The listing builds one solid part. Answer for the finished solid, in the listing's coordinates (mm). Face numbers are marked on the shaded views. Round coordinates to 2 decimals unless told otherwise and drop trailing zeros. Loops run counter-clockwise (first coordinate to the right, second up) from the corner with the lowest first, then second, coordinate; pieces in that order, holes last. Notation, with made-up numbers: M 73.5,17 L 86.5,17 A19 cw 86.5,23 Z; hole C 25.25,-19 d2. An arc over 180 degrees is marked long. Put each result on its own line as item: value. Start each with the question number.
(1) Section B-B, the plane z = 50 is taken. Determine the outline of the cut face in (x, y).
(2) Flat-ended cylindrical pins translate along their axes: P1, Ø10, axis at y = 1.5, z = 57.5, coming from the +X side (3 decimals); P2, Ø2.5, axis at x = 1.5, y = 12.5, coming from the +Z side; P3, Ø6, axis at x = -0.5, y = 7, coming from the +Z side; P4, Ø1, axis at y = 2, z = 89, coming from the -X side. Find the tip coordinate at first contact, or state that the pin passes through.
(3) Section D-D, the plane x = -20 is taken. Count the separate pieces of the cut face and the enclosed holes in it, then the cut area to 3 significant figures.
(4) Section A-A, the plane x = 1.5 is taken. Determine the outline of the cut face in (y, z), then the cut area to 3 significant figures.
(5) Straight lines are drawn through the part: line 1 (X direction, y = 11.5, z = 94); line 2 (Y direction, x = 0, z = 88.5); line 3 (Z direction, x = -23.5, y = 5.5). For each, find the intervals that lie inside material, in ascending order.
(6) Determine the mould class of the marked faces 1, 2 and 3 for opening direction X: released by +X, released by -X, zero draft, split by the parting line, or undercut.
(7) Section C-C, the plane y = -13 is taken. Determine the outline of the cut face in (x, z).
```python
from build123d import *

# Parameters (mm, degrees)
PAD_DEPTH       = 116
SKETCH001_R     = 1.75
POCKET_DEPTH    = 17.6055143834
SKETCH002_R     = 4
POCKET001_DEPTH = 14
SKETCH003_W     = 20
SKETCH003_H     = 16
POCKET002_DEPTH = 5
FILLET_R        = 2
FILLET001_R     = 2
FILLET002_R     = 0.5
FILLET003_R     = 0.5


with BuildPart() as part:
    # Sketch (on XY_Plane of Origin) → Pad (new body)
    with BuildSketch(Plane.XY):
        Polygon((10.1949841474, 13.6874291489), (-11.9050158526, 13.6874291489), (-27.9319746193, 13.6874291489), (-11.9050158526, -20.6824948412), (10.1949841474, -20.6824948412), (10.1949841474, -18.6824948412), (10.1949841474, -17.3125708511), (8.1949841474, -17.3125708511), (8.1949841474, -18.3125708511), (-9.9050158526, -18.3125708511), (-9.9050158526, 11.6874291489), (8.1949841474, 11.6874291489), (8.1949841474, 10.6874291489), (10.1949841474, 10.6874291489), align=None)
    extrude(amount=PAD_DEPTH)

    # Sketch001 (on Face10 of Pad) → Pocket (cut)
    with BuildSketch(Plane(origin=(-17.7005613893, -8.2539073295, 0), x_dir=(0.4226182617, -0.906307787, 0), z_dir=(-0.906307787, -0.4226182617, 0))):
        with Locations((-16, 109.75)):
            Circle(SKETCH001_R)
        with Locations((-16, 12.25)):
            Circle(SKETCH001_R)
    extrude(amount=-POCKET_DEPTH, mode=Mode.SUBTRACT)

    # Sketch002 (on Face12 of Pocket) → Pocket001 (cut)
    with BuildSketch(Plane(origin=(2.2382099255, 1.0436944288, 0), x_dir=(0.4226182617, -0.906307787, 0), z_dir=(-0.906307787, -0.4226182617, 0))):
        with Locations((-16, 109.75)):
            Circle(SKETCH002_R)
        with Locations((-16, 12.25)):
            Circle(SKETCH002_R)
    extrude(amount=POCKET001_DEPTH, mode=Mode.SUBTRACT)

    # Sketch003 (on Face11 of Pocket001) → Pocket002 (cut)
    with BuildSketch(Plane(origin=(0, 13.6874291489, 0), x_dir=(-1, 0, 0), z_dir=(0, 1, 0))):
        with Locations((-0.1949841474, 8)):
            Rectangle(SKETCH003_W, SKETCH003_H)
        with Locations((-0.1949841474, 108)):
            Rectangle(SKETCH003_W, SKETCH003_H)
    extrude(amount=-POCKET002_DEPTH, mode=Mode.SUBTRACT)

    # Fillet
    fillet_edges = [part.edges().sort_by_distance(p)[0] for p in [
        (-27.931975, 13.687429, 58),
        (-11.905016, -20.682495, 58),
    ]]
    fillet(fillet_edges, radius=FILLET_R)

    # Fillet001
    fillet001_edges = [part.edges().sort_by_distance(p)[0] for p in [
        (10.194984, -20.682495, 58),
        (10.194984, 13.687429, 58),
    ]]
    fillet(fillet001_edges, radius=FILLET001_R)

    # Fillet002
    fillet002_edges = [part.edges().sort_by_distance(p)[0] for p in [
        (8.194984, 10.687429, 58),
        (8.194984, -17.312571, 58),
    ]]
    fillet(fillet002_edges, radius=FILLET002_R)

    # Fillet003
    fillet003_edges = [part.edges().sort_by_distance(p)[0] for p in [
        (10.194984, 10.687429, 58),
        (10.194984, -17.312571, 58),
    ]]
    fillet(fillet003_edges, radius=FILLET003_R)


solid = part.part
```
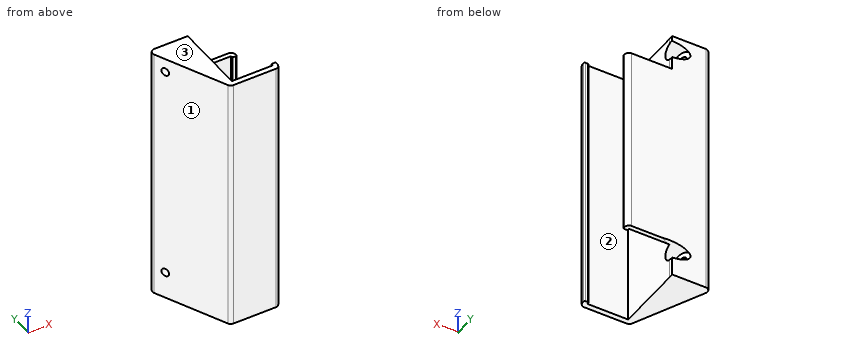
Recorded:
1. outline: M -26.61,10.84 L -12.44,-19.53 A2 ccw -10.63,-20.68 L 8.19,-20.68 A2 ccw 10.19,-18.68 L 10.19,-17.81 A0.5 ccw 9.69,-17.31 L 8.69,-17.31 A0.5 ccw 8.19,-17.81 L 8.19,-18.31 L -9.91,-18.31 L -9.91,11.69 L 8.19,11.69 L 8.19,11.19 A0.5 ccw 8.69,10.69 L 9.69,10.69 A0.5 ccw 10.19,11.19 L 10.19,11.69 A2 ccw 8.19,13.69 L -24.79,13.69 A2 ccw Z
2. P1: stops at x = -9.905
2. P2: stops at z = 100
2. P3: passes through
2. P4: stops at x = -22.72
3. separate pieces: 1
3. enclosed holes: 2
3. area: 1,950 mm²
4. outline: M -20.68,0 L -18.31,0 L -18.31,116 L -20.68,116 Z; M 11.69,16 L 13.69,16 L 13.69,100 L 11.69,100 Z
4. area: 443 mm²
5. line 1: x = -26.78 to -9.91, 8.19 to 10.19
5. line 2: y = -20.68 to -18.31, 11.69 to 13.69
5. line 3: z = 0 to 10.88, 13.62 to 108.38, 111.12 to 116
6. face 1: released by -X
6. face 2: undercut
6. face 3: zero draft
7. outline: M -15.49,0 L -9.91,0 L -9.91,116 L -15.49,116 Z
